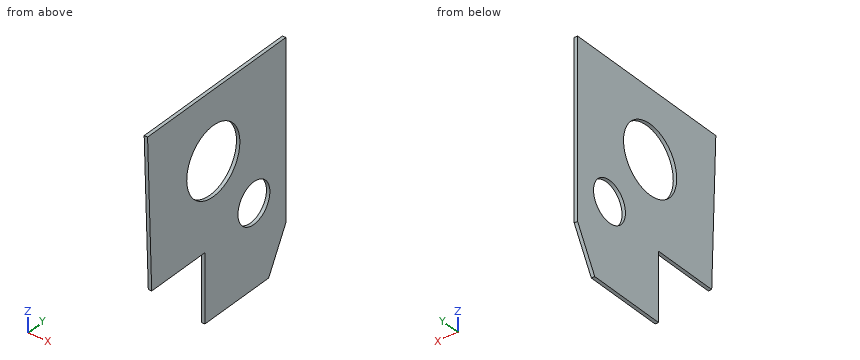
```python
from build123d import *

# Parameters (mm, degrees)
BOSS_EXTRUDE1_DEPTH = 3.175
SKETCH3_R           = 31.75
SKETCH3_R_2         = 19.05
CUT_EXTRUDE3_DEPTH  = 349.186809908


with BuildPart() as part:
    # Sketch2 → Boss-Extrude1 (new body)
    with BuildSketch(Plane(origin=(0, 0, 0), x_dir=(0, 0, -1), z_dir=(1, 0, 0))):
        Polygon((-337.942750929, 83.777509294), (-172.842750929, 83.777509294), (-134.742750929, 63.287546468), (-134.742750929, -12.912453532), (-198.242750929, -12.912453532), (-198.242750929, -76.412453532), (-337.942750929, -81.322490706), align=None)
    extrude(amount=BOSS_EXTRUDE1_DEPTH)

    # Sketch3 → Cut-Extrude3 (cut, through all)
    with BuildSketch(Plane(origin=(3.175, 0, 0), x_dir=(0, 0, -1), z_dir=(1, 0, 0))):
        with Locations((-274.442750929, -2.843604756)):
            Circle(SKETCH3_R)
        with Locations((-210.942750929, 45.677509294)):
            Circle(SKETCH3_R_2)
    extrude(amount=-CUT_EXTRUDE3_DEPTH, mode=Mode.SUBTRACT)


solid = part.part
```
Part model, mm, in its own coordinate system. Round coordinates to 2 decimals unless told otherwise and drop trailing zeros. Write each loop counter-clockwise with the first axis right and the second up, starting at its lowest first coordinate (ties: lowest second). Pieces come first, ordered by that corner, then holes. Notation, with made-up numbers: (48.5, 25.5) -> (93.5, 25.5) arc R16 cw to (93.5, 30.5) -> close; hole circle Ø9 at (11.25, 47.25). An arc over 180 degrees is marked (long way). Return JSON: item names as keys, results as strings. Group by question number.
Q1. Saw through at C-C on x = 1.85. Write the cut outline in (y, z), plus the area to 3 significant figures.
Q2. Probe L1, parallel to Z at x = 1.45, y = -48; L2, parallel to Z at x = 0.4, y = 5; L3, parallel to Z at x = 1.15, y = 54.5. List the from-to ranges inside material, lowest first. Write a range as [from, to].
Q3. Saw through at B-B on y = -9.5. Write the cut outline in (x, z) (3 decimals), plus the area to 3 significant figures.
Q4. Pin check, flat tip, straight feed: pin 1 (1.6 mm diameter, centred on x = 1, z = 182, fed in from -Y). Stop position of the tip, or through.
Q5. Saw through at A-A on z = 293. Write the cut outline in (x, y) (1 decimal), plus the area to 3 significant figures.
Q6. Saw through at D-D on z = 180.5. Write the cut outline in (x, y) (1 decimal), plus the area to 3 significant figures.
Answer:
{
 "1": {"outline": "(-81.32, 337.94) -> (-76.41, 198.24) -> (-12.91, 198.24) -> (-12.91, 134.74) -> (63.29, 134.74) -> (83.78, 172.84) -> (83.78, 337.94) -> close; hole circle Ø63.5 at (-2.84, 274.44); hole circle Ø38.1 at (45.68, 210.94)", "area": "24,200 mm2"},
 "2": {"L1": "[198.24, 337.94]", "L2": "[134.74, 243.68], [305.21, 337.94]", "L3": "[134.74, 194.06], [227.83, 337.94]"},
 "3": {"outline": "(0, 134.743) -> (3.175, 134.743) -> (3.175, 243.398) -> (0, 243.398) -> close; (0, 305.487) -> (3.175, 305.487) -> (3.175, 337.943) -> (0, 337.943) -> close", "area": "448 mm2"},
 "4": {"pin 1": "y = -12.91"},
 "5": {"outline": "(0, -79.7) -> (3.2, -79.7) -> (3.2, -28.6) -> (0, -28.6) -> close; (0, 22.9) -> (3.2, 22.9) -> (3.2, 83.8) -> (0, 83.8) -> close", "area": "356 mm2"},
 "6": {"outline": "(0, -12.9) -> (3.2, -12.9) -> (3.2, 83.8) -> (0, 83.8) -> close", "area": "307 mm2"}
}
